CAD build for the part. Positions are in the model's coordinates, mm. Coordinates: 2 decimals unless noted, no trailing zeros. Loops run counter-clockwise (first coordinate to the right, second up) from the corner with the lowest first, then second, coordinate; pieces in that order, holes last. Notation, with made-up numbers: (8.25, 46) -> (43.25, 46) arc R29 cw to (43.25, 72) -> close; hole circle Ø8 at (-8.5, -17.75). An arc over 180 degrees is marked (long way). Answer as a JSON object with one key per item and string values. Group by question number.
from build123d import *

# Parameters (mm, degrees)
SKETCH1_R           = 0.7
SKETCH1_W           = 2.4
SKETCH1_H           = 5.125
BOSS_EXTRUDE1_DEPTH = 0.8


with BuildPart() as part:
    # Sketch1 → Boss-Extrude1 (new body)
    with BuildSketch(Plane.XY):
        Polygon((0, 30), (2.4, 30), (2.4, 31), (6.05, 31), (6.05, 15), (2.4, 15), (2.4, 16), (0, 16), (0, 3.7), (-3.7, 0), (-36.3, 0), (-40, 3.7), (-40, 16), (-42.4, 16), (-42.4, 15), (-46.05, 15), (-46.05, 31), (-42.4, 31), (-42.4, 30), (-40, 30), (-40, 42.3), (-36.3, 46), (-3.7, 46), (0, 42.3), align=None)
        with Locations((4.21811613, 23)):
            Circle(SKETCH1_R, mode=Mode.SUBTRACT)
        with Locations((-44.262582218, 23)):
            Circle(SKETCH1_R, mode=Mode.SUBTRACT)
        with Locations((1.2, 19.8125)):
            Rectangle(SKETCH1_W, SKETCH1_H, mode=Mode.SUBTRACT)
        with Locations((1.2, 26.1875)):
            Rectangle(SKETCH1_W, SKETCH1_H, mode=Mode.SUBTRACT)
        with Locations((-41.2, 26.1875)):
            Rectangle(SKETCH1_W, SKETCH1_H, mode=Mode.SUBTRACT)
        with Locations((-41.2, 19.8125)):
            Rectangle(SKETCH1_W, SKETCH1_H, mode=Mode.SUBTRACT)
    extrude(amount=BOSS_EXTRUDE1_DEPTH)


solid = part.part
Item 1: Flat gauge pins, fed straight in: P1, Ø10, axis at x = -1, y = 10.5, coming from the -Z side; P2, Ø1.1, axis at x = -44.26, y = 23, coming from the -Z side. Where does each tip first touch, or does it go through?
Item 2: Pull direction X, two halves, no side cores. Call faces 1 (the flat face through (-38.2, 44.1, 0.4)), 2 (the flat face through (-20, 23, 0.8)), 3 (the cylindrical face through (-43.9, 23.6, 0.4)): +X half, -X half, draft (parallel to the pull), parting line (faces both ways), or undercut.
Item 3: Band-saw the part on B-B, the plane x = -3. List the corners of the cut face in (y, z), and give its area (3 significant figures).
Item 4: Drill centre lines: L1, parallel to X at y = 25, z = 0.3; L2, parallel to X at y = 37, z = 0.25; L3, parallel to Y at x = -44, z = 0.2. Where is each one in solid material? Low to high.
Item 5: Band-saw the part on D-D, the plane y = 36.5. List the corners of the cut face in (x, z), and give its area (3 significant figures).
Item 6: Band-saw the part on A-A, the plane y = 23. List the corners of the cut face in (x, z).
Item 7: Band-saw the part on C-C, the plane z = 0.15. Count the separate pieces of the cut face and the enclosed holes in it, and give its area (3 significant figures).
Reply:
{
 "1": {"P1": "z = 0", "P2": "through"},
 "2": {"face 1": "-X half", "face 2": "draft", "face 3": "undercut"},
 "3": {"outline": "(0.7, 0) -> (45.3, 0) -> (45.3, 0.8) -> (0.7, 0.8) -> close", "area": "35.7 mm²"},
 "4": {"L1": "-46.05 to -42.4, -40 to 0, 2.4 to 6.05", "L2": "-40 to 0", "L3": "15 to 22.35, 23.65 to 31"},
 "5": {"outline": "(-40, 0) -> (0, 0) -> (0, 0.8) -> (-40, 0.8) -> close", "area": "32.0 mm²"},
 "6": {"outline": "(-46.05, 0) -> (-44.96, 0) -> (-44.96, 0.8) -> (-46.05, 0.8) -> close; (-43.56, 0) -> (3.52, 0) -> (3.52, 0.8) -> (-43.56, 0.8) -> close; (4.92, 0) -> (6.05, 0) -> (6.05, 0.8) -> (4.92, 0.8) -> close"},
 "7": {"separate pieces": "1", "enclosed holes": "6", "area": "1,940 mm²"}
}
